Verification items for this drawing (mm, ordinates from the low corner). Coordinates: 2 decimals unless noted, no trailing zeros. Order: outer loops, then holes, each group sorted by start corner. A loop starts at its lowest first (then second) coordinate and runs counter-clockwise, first axis right, second up. Notation, with made-up numbers: (26.25, 89) -> (48.25, 89) arc R31 ccw to (48.25, 118) -> close; hole circle Ø1 at (3.25, -2). An arc over 180 degrees is marked (long way). Answer in a Markdown table with one row per item. Add a question column.
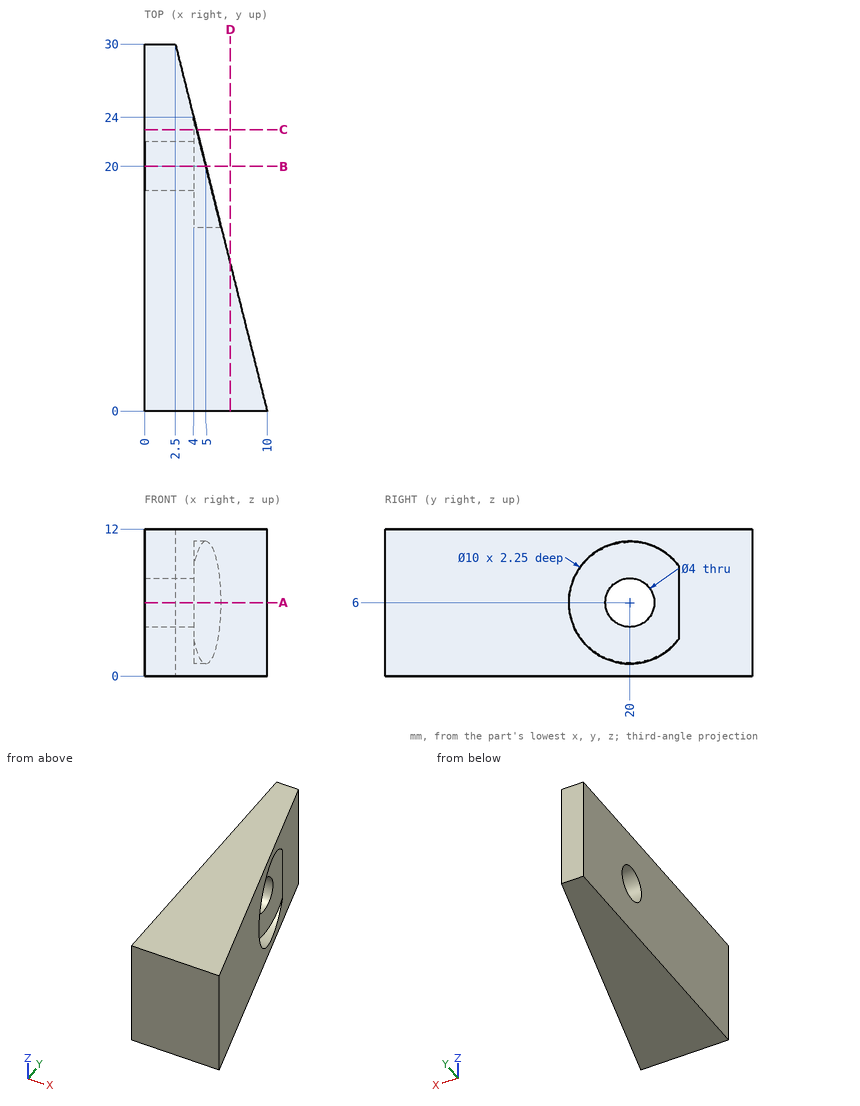
(1) Cross-section at C-C (y = 23). Enter the section's corners in (x, z).
(2) Cross-section at D-D (x = 7). Enter the section's corners in (y, z).
(3) Cross-section at A-A (z = 6). Enter the section's corners in (x, y).
(4) Cross-section at B-B (y = 20). Enter the section's corners in (x, z).
(5) Scan lines: line 1 along Z through (x, y) = (4.5, 20); line 2 along X through (y, z) = (21.75, 10.5); line 3 along Y through (x, z) = (1.15, 6). Record each from-to range of solid material in increasing order.
(6) Go/stop test with flat-tipped pins: P1, Ø4.5, axis at y = 18, z = 4, coming from the +X side; P2, Ø1, axis at x = 7.5, y = 17.5, coming from the +Z side. Record where each tip stops, or that it passes through.
Checks:
| question | item | result |
|---|---|---|
| 1 | outline | (0, 0) -> (4.25, 0) -> (4.25, 2) -> (4, 2) -> (4, 10) -> (4.25, 10) -> (4.25, 12) -> (0, 12) -> close |
| 2 | outline | (0, 0) -> (12, 0) -> (12, 12) -> (0, 12) -> close |
| 3 | outline | (0, 0) -> (10, 0) -> (6.25, 15) -> (4, 15) -> (4, 18) -> (0, 18) -> close; (0, 22) -> (4, 22) -> (4, 24) -> (2.5, 30) -> (0, 30) -> close |
| 4 | outline | (0, 0) -> (5, 0) -> (5, 1) -> (4, 1) -> (4, 4) -> (0, 4) -> close; (0, 8) -> (4, 8) -> (4, 11) -> (5, 11) -> (5, 12) -> (0, 12) -> close |
| 5 | line 1 | 0 to 1, 11 to 12 |
| 5 | line 2 | 0 to 4 |
| 5 | line 3 | 0 to 18, 22 to 30 |
| 6 | P1 | x = 6.01 |
| 6 | P2 | through |
